Autodesk Inventor part; units mm, degrees
ref_plane "YZ Plane" through (0, 0, 0) normal (1, 0, 0) x (0, 1, 0)
ref_plane "XZ Plane" through (0, 0, 0) normal (0, 1, 0) x (-1, 0, 0)
ref_plane "XY Plane" through (0, 0, 0) normal (0, 0, 1) x (1, 0, 0)
sketch "Sketch1" plane through (0, 0, 0) normal (0, 1, 0) x (-1, 0, 0)
  line L0 (25, -65.5) -> (-25, -65.5)
  line L1 (-25, 65.5) -> (25, 65.5)
  circle A0 centre (0, 0) radius 4
  circle A1 centre (-6, -25) radius 1
  circle A2 centre (-6, 25) radius 1
  line L2 (-25, 65.5) -> (-10, 65.5)
  line L3 (-10, 50.6) -> (-25, 50.6)
  line L4 (-25, 50.6) -> (-25, 65.5)
  line L5 (-25, 65.5) -> (-10, 65.5)
  line L6 (-10, 40.6) -> (-25, 40.6)
  line L7 (-25, -65.5) -> (-10, -65.5)
  line L8 (-10, -40.6) -> (-25, -40.6)
  line L9 (-25, -65.5) -> (-10, -65.5)
  line L10 (-10, -50.6) -> (-25, -50.6)
  line L11 (-25, -50.6) -> (-25, -65.5)
  line L12 (25, -65.5) -> (10, -65.5)
  line L13 (10, -40.6) -> (25, -40.6)
  line L14 (25, -65.5) -> (10, -65.5)
  line L15 (10, -50.6) -> (25, -50.6)
  line L16 (25, -50.6) -> (25, -65.5)
  line L17 (25, 65.5) -> (10, 65.5)
  line L18 (10, 40.6) -> (25, 40.6)
  line L19 (25, 65.5) -> (10, 65.5)
  line L20 (10, 50.6) -> (25, 50.6)
  line L21 (25, 50.6) -> (25, 65.5)
  line L22 (-10, 50.6) -> (-10, 40.6)
  line L23 (-25, 40.6) -> (-25, -40.6)
  line L24 (-10, -40.6) -> (-10, -50.6)
  line L25 (10, -40.6) -> (10, -50.6)
  line L26 (25, -40.6) -> (25, 40.6)
  line L27 (10, 40.6) -> (10, 50.6)
  dimension "d0" = 50
  dimension "d1" = 131
  dimension "d4" = 8
  dimension "d10" = 2
  dimension "d18" = 14.9
  dimension "d19" = 15
  dimension "d20" = 24.9
  dimension "d21" = 15
  dimension "d22" = 24.9
  dimension "d24" = 14.9
  dimension "d25" = 15
  dimension "d26" = 24.9
  dimension "d28" = 14.9
  dimension "d29" = 15
  dimension "d30" = 24.9
  dimension "d32" = 14.9
extrude "Extrusion1" add sketch "Sketch1" along normal blind 10 contours L0 L11 L10 L24 L8 L23 L6 L22 L3 L4 L1 L21 L20 L27 L18 L26 L13 L25 L15 L16 | A0 | A1 | A2
extrude "Extrusion2" cut sketch "Sketch1" along normal blind 10 contours A0 | A1 | A2
sketch "Sketch3" plane through (-25, 0, -40.6) normal (-1, 0, 0) x (0, 0, 1)
  circle A0 centre (40.6, 5) radius 1.25
  point P0 (40.6, 0)
  dimension "d34" = 2.5
extrude "Extrusion4" cut sketch "Sketch3" against normal blind 10
properties part number "predni_komatex(0)"
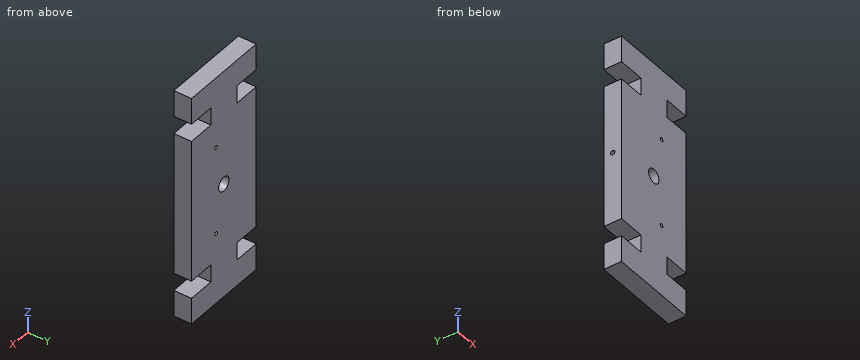
The listing builds one solid part. Answer for the finished solid, in the listing's coordinates (mm). Give positions to 0.01 mm unless a question says otherwise; leave off trailing zeros. Order: outer loops, then holes, each group sorted by start corner. A loop starts at its lowest first (then second) coordinate and runs counter-clockwise, first axis right, second up. Notation, with made-up numbers: (-9.5, 35) -> (46.5, 35) arc R25 cw to (46.5, 74) -> close; hole circle Ø9 at (-39.75, 44.5). An arc over 180 degrees is marked (long way). Write each question's results on one line, items separated by ' | '.
Q1. The part is cut by section D-D, the plane y = 5. Give the vertices of the cut face in (x, z).
Checked values:
outline: (-25, -65.5) -> (25, -65.5) -> (25, -50.6) -> (10, -50.6) -> (10, -40.6) -> (25, -40.6) -> (25, 40.6) -> (10, 40.6) -> (10, 50.6) -> (25, 50.6) -> (25, 65.5) -> (-25, 65.5) -> (-25, 50.6) -> (-10, 50.6) -> (-10, 40.6) -> (-25, 40.6) -> (-25, 1.25) -> (-15, 1.25) -> (-15, -1.25) -> (-25, -1.25) -> (-25, -40.6) -> (-10, -40.6) -> (-10, -50.6) -> (-25, -50.6) -> close; hole circle Ø8 at (0, 0); hole circle Ø2 at (6, -25); hole circle Ø2 at (6, 25)
Q2. The part is cut by section C-C, the plane x = -17. Give the vertices of the cut face in (y, z), and give its area (3 significant figures).
Checked values:
outline: (0, -65.5) -> (10, -65.5) -> (10, -50.6) -> (0, -50.6) -> close; (0, -40.6) -> (10, -40.6) -> (10, 40.6) -> (0, 40.6) -> close; (0, 50.6) -> (10, 50.6) -> (10, 65.5) -> (0, 65.5) -> close; hole circle Ø2.5 at (5, 0) | area: 1,110 mm^2
Q3. Straight lines are drawn through the part: probe 1 along Z at (x, y) = (6, 2.5); probe 2 along Z at (x, y) = (-20, 8.5); probe 3 along Z at (x, y) = (0, 6.75). For each, find the intervals that lie inside material, in ascending order. Write a range as from..to.
Checked values:
probe 1: z = -65.5..-26, -24..24, 26..65.5 | probe 2: z = -65.5..-50.6, -40.6..40.6, 50.6..65.5 | probe 3: z = -65.5..-4, 4..65.5
Q4. Each of these flat-tipped pins is pushed along its axis until it touches: P1, Ø1.2, axis at x = 6, z = 25, coming from the +Y side; P2, Ø1.5, axis at y = 7.5, z = 48.5, coming from the +X side; P3, Ø3, axis at y = 6.5, z = 46, coming from the -X side; P4, Ø1.2, axis at y = 5, z = 0, coming from the -X side. Where does it stop, or does it pass through?
Checked values:
P1: passes through | P2: stops at x = 10 | P3: stops at x = -10 | P4: stops at x = -15
Q5. The part is cut by section B-B, the plane x = 0. Give the vertices of the cut face in (y, z), and give its area (3 significant figures).
Checked values:
outline: (0, -65.5) -> (10, -65.5) -> (10, -4) -> (0, -4) -> close; (0, 4) -> (10, 4) -> (10, 65.5) -> (0, 65.5) -> close | area: 1,230 mm^2
Q6. The part is cut by section A-A, the plane z = 0. Give the vertices of the cut face in (x, y), and give its area (3 significant figures).
Checked values:
outline: (-25, 0) -> (-4, 0) -> (-4, 10) -> (-25, 10) -> (-25, 6.25) -> (-15, 6.25) -> (-15, 3.75) -> (-25, 3.75) -> close; (4, 0) -> (25, 0) -> (25, 10) -> (4, 10) -> close | area: 395 mm^2
